Autodesk Fusion 360 part; units mm, degrees
sketch "Sketch2" plane through (0, 0, 0) normal (0, 0, 1) x (1, 0, 0)
  line L0 (-46, 50) -> (126, 50)
  line L1 (130, 46) -> (130, -76)
  line L2 (126, -80) -> (-46, -80)
  line L3 (-50, -76) -> (-50, 46)
  circle A0 centre (-45, 45) radius 2
  line L4 (40, -80) -> (40, 50) construction
  line L5 (-50, -15) -> (130, -15) construction
  arc A1 (-46, 50) -> (-50, 46) centre (-46, 46) ccw
  circle A2 centre (125, 45) radius 2
  arc A3 (130, 46) -> (126, 50) centre (126, 46) ccw
  circle A4 centre (125, -75) radius 2
  arc A5 (126, -80) -> (130, -76) centre (126, -76) ccw
  circle A6 centre (-45, -75) radius 2
  arc A7 (-50, -76) -> (-46, -80) centre (-46, -76) ccw
  point P0 (-50, 50)
  point P1 (130, 50)
  dimension "d3" = 4
  dimension "d4" = 5
  dimension "d5" = 5
  dimension "d6" = 4
  dimension "d63" = 180
  dimension "d64" = 130
extrude "Extrude1" add sketch "Sketch2" along normal blind 6
sketch "Sketch3" plane through (0, 0, 0) normal (0, 0, -1) x (1, 0, 0)
  circle A0 centre (125, 75) radius 2
  circle A1 centre (-45, 75) radius 2
  circle A2 centre (-45, -45) radius 2
  circle A3 centre (125, -45) radius 2
  arc A4 (-50, -46) -> (-46, -50) centre (-46, -46) ccw
  line L0 (-46, -50) -> (126, -50)
  arc A5 (126, -50) -> (130, -46) centre (126, -46) ccw
  line L1 (130, -46) -> (130, 76)
  arc A6 (130, 76) -> (126, 80) centre (126, 76) ccw
  line L2 (126, 80) -> (-46, 80)
  arc A7 (-46, 80) -> (-50, 76) centre (-46, 76) ccw
  line L3 (-50, 76) -> (-50, -46)
  line L4 (40, 80) -> (40, -50) construction
  line L5 (130, 15) -> (-50, 15) construction
  line L6 (119.9494, -39.9494) -> (-39.9494, -39.9494) construction
  line L7 (-39.9494, -39.9494) -> (-39.9494, 69.9494) construction
  line L8 (-39.9494, 69.9494) -> (119.9494, 69.9494) construction
  line L9 (119.9494, 69.9494) -> (119.9494, -39.9494) construction
  line L10 (119.9494, -39.9494) -> (-39.9494, 69.9494) construction
  line L11 (-39.9494, -39.9494) -> (119.9494, 69.9494) construction
  line L12 (108.2459, -41.3839) -> (-28.2459, -41.3839)
  line L13 (-41.3839, -28.2459) -> (-41.3839, 58.2459)
  line L14 (-28.2459, 71.3839) -> (108.2459, 71.3839)
  line L15 (121.3839, 58.2459) -> (121.3839, -28.2459)
  line L16 (95.6336, -23.5438) -> (-41.3839, 71.3839) construction
  line L17 (-38.6963, -33.1786) -> (83.6146, 41.7012) construction
  line L18 (-38.5149, -28.2459) -> (-38.5149, 58.2459)
  line L19 (-28.2459, 68.5149) -> (108.2459, 68.5149)
  line L20 (118.5149, 58.2459) -> (118.5149, -28.2459)
  line L21 (104.513, -28.9713) -> (-38.5149, 68.5149) construction
  line L22 (-36.0332, -30.305) -> (80.8211, 39.3236) construction
  arc A8 (-28.2459, 68.5149) -> (-38.5149, 58.2459) centre (-28.2459, 58.2459) ccw
  arc A9 (-28.2459, 71.3839) -> (-41.3839, 58.2459) centre (-28.2459, 58.2459) ccw
  arc A10 (118.5149, 58.2459) -> (108.2459, 68.5149) centre (108.2459, 58.2459) ccw
  arc A11 (121.3839, 58.2459) -> (108.2459, 71.3839) centre (108.2459, 58.2459) ccw
  arc A12 (-38.5149, -28.2459) -> (-28.2459, -38.5149) centre (-28.2459, -28.2459) ccw
  arc A13 (-41.3839, -28.2459) -> (-28.2459, -41.3839) centre (-28.2459, -28.2459) ccw
  arc A14 (108.2459, -38.5149) -> (118.5149, -28.2459) centre (108.2459, -28.2459) ccw
  arc A15 (108.2459, -41.3839) -> (121.3839, -28.2459) centre (108.2459, -28.2459) ccw
  line L23 (108.2459, -38.5149) -> (-28.2459, -38.5149)
  point P0 (40, 15)
  point P1 (40, 15)
  point P2 (40, 15)
  point P3 (40, 15)
  point P4 (40, 15)
  dimension "d25" = 159.8988
  dimension "d27" = 109.8988
  dimension "d28" = 1.4345
  dimension "d29" = 1.4345
  dimension "d30" = 1.4345
  dimension "d31" = 1.4345
  dimension "d44" = 10.269
  dimension "d45" = 13.138
extrude "Extrude4" add sketch "Sketch3" along normal blind 1.424 contours L12 L13 L14 L15 A9 A11 A13 A15
draft "Draft3" angle 10 neutral plane through (0, 0, -1.424) pull (0, 0, -1) 16 faces at (62.7486, -68.5149, -0.9493) (117.7793, -62.0625, -0.9493) (118.5149, -29.4153, -0.4747) (115.6779, 35.3323, -0.9493) (62.7486, 38.5149, -0.4747) (-32.9514, 37.3734, -0.9493) (-38.5149, -29.4153, -0.9493) (-35.6779, -65.3323, -0.9493) (-41.3839, -0.5847, -0.4747) (-33.1288, 40.4428, -0.9493) (17.2514, 41.3839, -0.9493) (116.3673, 38.5731, -0.9493) (121.3839, -29.4153, -0.9493) (119.6238, -64.8149, -0.9493) (62.7486, -71.3839, -0.9493) (-38.9478, -65.8667, -0.9493)
sketch "Sketch5" plane through (0, 0, -1.424) normal (0, 0, -1) x (1, 0, 0)
  line L0 (-28.2459, 68.5149) -> (108.2459, 68.5149)
  line L1 (118.5149, 58.2459) -> (118.5149, -28.2459)
  line L2 (108.2459, -38.5149) -> (-28.2459, -38.5149)
  line L3 (-38.5149, -28.2459) -> (-38.5149, 58.2459)
  line L4 (108.2459, 71.3839) -> (-28.2459, 71.3839)
  line L5 (-41.3839, 58.2459) -> (-41.3839, -28.2459)
  line L6 (-28.2459, -41.3839) -> (108.2459, -41.3839)
  line L7 (121.3839, -28.2459) -> (121.3839, 58.2459)
  line L8 (40, 71.3839) -> (40, -41.3839) construction
  line L9 (121.3839, 15) -> (-41.3839, 15) construction
  line L10 (119.9494, -39.9494) -> (-39.9494, -39.9494) construction
  line L11 (-39.9494, -39.9494) -> (-39.9494, 69.9494) construction
  line L12 (-39.9494, 69.9494) -> (119.9494, 69.9494) construction
  line L13 (119.9494, 69.9494) -> (119.9494, -39.9494) construction
  line L14 (119.9494, -39.9494) -> (-39.9494, 69.9494) construction
  line L15 (-39.9494, -39.9494) -> (119.9494, 69.9494) construction
  line L16 (108.2459, -40.8839) -> (-28.2459, -40.8839)
  line L17 (-40.8839, -28.2459) -> (-40.8839, 58.2459)
  line L18 (-28.2459, 70.8839) -> (108.2459, 70.8839)
  line L19 (120.8839, 58.2459) -> (120.8839, -28.2459)
  line L20 (98.0985, -25.1411) -> (-40.8839, 70.8839) construction
  line L21 (-40.8839, -40.8839) -> (98.0985, 55.1411) construction
  line L22 (108.2459, -39.0149) -> (-28.2459, -39.0149)
  line L23 (-39.0149, -28.2459) -> (-39.0149, 58.2459)
  line L24 (119.0149, 58.2459) -> (119.0149, -28.2459)
  line L25 (97.1479, -24.0666) -> (-39.0149, 69.0149) construction
  line L26 (-39.0149, -39.0149) -> (97.1479, 54.0666) construction
  arc A0 (118.5149, 58.2459) -> (108.2459, 68.5149) centre (108.2459, 58.2459) ccw
  arc A1 (108.2459, -38.5149) -> (118.5149, -28.2459) centre (108.2459, -28.2459) ccw
  arc A2 (-38.5149, -28.2459) -> (-28.2459, -38.5149) centre (-28.2459, -28.2459) ccw
  arc A3 (-28.2459, 68.5149) -> (-38.5149, 58.2459) centre (-28.2459, 58.2459) ccw
  arc A4 (-41.3839, -28.2459) -> (-28.2459, -41.3839) centre (-28.2459, -28.2459) ccw
  arc A5 (108.2459, -41.3839) -> (121.3839, -28.2459) centre (108.2459, -28.2459) ccw
  arc A6 (121.3839, 58.2459) -> (108.2459, 71.3839) centre (108.2459, 58.2459) ccw
  arc A7 (-28.2459, 71.3839) -> (-41.3839, 58.2459) centre (-28.2459, 58.2459) ccw
  arc A8 (-28.2459, 69.0149) -> (-39.0149, 58.2459) centre (-28.2459, 58.2459) ccw
  arc A9 (-28.2459, 70.8839) -> (-40.8839, 58.2459) centre (-28.2459, 58.2459) ccw
  arc A10 (119.0149, 58.2459) -> (108.2459, 69.0149) centre (108.2459, 58.2459) ccw
  arc A11 (120.8839, 58.2459) -> (108.2459, 70.8839) centre (108.2459, 58.2459) ccw
  line L27 (-28.2459, 69.0149) -> (108.2459, 69.0149)
  arc A12 (108.2459, -39.0149) -> (119.0149, -28.2459) centre (108.2459, -28.2459) ccw
  arc A13 (108.2459, -40.8839) -> (120.8839, -28.2459) centre (108.2459, -28.2459) ccw
  arc A14 (-39.0149, -28.2459) -> (-28.2459, -39.0149) centre (-28.2459, -28.2459) ccw
  arc A15 (-40.8839, -28.2459) -> (-28.2459, -40.8839) centre (-28.2459, -28.2459) ccw
  point P0 (40, 15)
  point P1 (40, 15)
  point P2 (40, 15)
  dimension "d36" = 159.8988
  dimension "d37" = 109.8988
  dimension "d38" = 0.9345
  dimension "d39" = 0.9345
  dimension "d40" = 0.9345
  dimension "d41" = 0.9345
  dimension "d50" = 10.769
  dimension "d51" = 12.638
extrude "Extrude6" cut sketch "Sketch5" against normal blind 1.424 contours L16 L17 L18 L19 A9 A11 A13 A15
extrude "Extrude7" cut 1 faces at (17.2514, 2.7546, 0) along direction (0, 0, 1) blind 0.5
sketch "Sketch6" plane through (0, 0, 0.5) normal (0, 0, -1) x (1, 0, 0)
  line L0 (108.2459, 68.2638) -> (-28.2459, 68.2638)
  arc A0 (-28.2459, 68.2638) -> (-38.2638, 58.2459) centre (-28.2459, 58.2459) ccw
  line L1 (-38.2638, 58.2459) -> (-38.2638, -28.2459)
  arc A1 (-38.2638, -28.2459) -> (-28.2459, -38.2638) centre (-28.2459, -28.2459) ccw
  line L2 (-28.2459, -38.2638) -> (108.2459, -38.2638)
  arc A2 (108.2459, -38.2638) -> (118.2638, -28.2459) centre (108.2459, -28.2459) ccw
  line L3 (118.2638, -28.2459) -> (118.2638, 58.2459)
  arc A3 (118.2638, 58.2459) -> (108.2459, 68.2638) centre (108.2459, 58.2459) ccw
  line L4 (40, 68.2638) -> (40, -38.2638) construction
  line L5 (-38.2638, 15) -> (118.2638, 15) construction
  line L6 (96, -27.5) -> (-16, -27.5)
  line L7 (-20, -23.5) -> (-20, 53.5)
  line L8 (-16, 57.5) -> (96, 57.5)
  line L9 (100, 53.5) -> (100, -23.5)
  line L10 (100, -27.5) -> (-20, 57.5) construction
  line L11 (-20, -27.5) -> (100, 57.5) construction
  arc A4 (-16, 57.5) -> (-20, 53.5) centre (-16, 53.5) ccw
  arc A5 (100, 53.5) -> (96, 57.5) centre (96, 53.5) ccw
  arc A6 (96, -27.5) -> (100, -23.5) centre (96, -23.5) ccw
  arc A7 (-20, -23.5) -> (-16, -27.5) centre (-16, -23.5) ccw
  point P0 (40, 15)
  dimension "d58" = 120
  dimension "d59" = 85
  dimension "d68" = 4
  dimension "d69" = 4
  dimension "d70" = 4
  dimension "d71" = 4
extrude "Extrude8" cut sketch "Sketch6" against normal blind 1.1 contours L6 L7 L8 L9 A4 A5 A6 A7
sketch "Sketch7" plane through (0, 0, 1.6) normal (0, 0, -1) x (1, 0, 0)
  line L0 (96, 57.5) -> (-16, 57.5)
  line L1 (-20, 53.5) -> (-20, -23.5)
  line L2 (-16, -27.5) -> (96, -27.5)
  line L3 (100, -23.5) -> (100, 53.5)
  line L4 (40, 57.5) -> (40, -27.5) construction
  line L5 (100, 15) -> (-20, 15) construction
  line L6 (91, -22.5) -> (-11, -22.5)
  line L7 (-15, -18.5) -> (-15, 48.5)
  line L8 (-11, 52.5) -> (91, 52.5)
  line L9 (95, 48.5) -> (95, -18.5)
  line L10 (95, -22.5) -> (-15, 52.5) construction
  line L11 (-15, -22.5) -> (95, 52.5) construction
  arc A0 (-16, 57.5) -> (-20, 53.5) centre (-16, 53.5) ccw
  arc A1 (-20, -23.5) -> (-16, -27.5) centre (-16, -23.5) ccw
  arc A2 (96, -27.5) -> (100, -23.5) centre (96, -23.5) ccw
  arc A3 (100, 53.5) -> (96, 57.5) centre (96, 53.5) ccw
  arc A4 (-11, 52.5) -> (-15, 48.5) centre (-11, 48.5) ccw
  arc A5 (95, 48.5) -> (91, 52.5) centre (91, 48.5) ccw
  arc A6 (91, -22.5) -> (95, -18.5) centre (91, -18.5) ccw
  arc A7 (-15, -18.5) -> (-11, -22.5) centre (-11, -18.5) ccw
  point P0 (40, 15)
  dimension "d62" = 110
  dimension "d65" = 75
  dimension "d72" = 4
  dimension "d73" = 4
  dimension "d74" = 4
  dimension "d75" = 4
extrude "Extrude9" cut sketch "Sketch7" against normal blind 8.4 contours L6 L7 L8 L9 A4 A5 A6 A7
equation "ORingDiameter = 1.78 mm"
equation "ORingInnerDiameter = 170 mm"
equation "d25 = ( ORingPerimeter - 100 mm ) / 4 + 50 mm"
equation "ORingPerimeter = 2 * 3.1412 * ( ( ORingInnerDiameter / 2 ) + ORingDiameter / 2 )"
equation "d27 = ( ORingPerimeter - 100 mm ) / 4"
equation "d28 = ( ( ORingDiameter * 1.05 ) / 2 ) + 0.5 mm"
equation "d29 = ( ( ORingDiameter * 1.05 ) / 2 ) + 0.5 mm"
equation "d30 = ( ( ORingDiameter * 1.05 ) / 2 ) + 0.5 mm"
equation "d31 = ( ( ORingDiameter * 1.05 ) / 2 ) + 0.5 mm"
equation "d32 = ORingDiameter * 0.8"
equation "d36 = ( ORingPerimeter - 100 mm ) / 4 + 50 mm"
equation "d37 = ( ORingPerimeter - 100 mm ) / 4"
equation "d38 = ( ORingDiameter * 1.05 ) / 2"
equation "d39 = ( ORingDiameter * 1.05 ) / 2"
equation "d40 = ( ORingDiameter * 1.05 ) / 2"
equation "d41 = ( ORingDiameter * 1.05 ) / 2"
equation "d44 = ( ORingDiameter ) * 6 + ORingDiameter * 0.05 - 0.5 mm"
equation "d45 = ( ORingDiameter ) * 6 + ( ORingDiameter * 1.1 ) + 0.5 mm"
equation "d50 = ( ORingDiameter ) * 6 + ORingDiameter * 0.05 - 0.0 mm"
equation "d51 = ( ORingDiameter ) * 6 + ORingDiameter * 1.1 + 0 mm"
equation "d52 = -( ORingDiameter * 0.8 )"
equation "PanelWidth = 85 mm"
equation "PanelLength = 120 mm"
equation "d58 = PanelLength"
equation "d59 = PanelWidth"
equation "d62 = PanelLength - 10 mm"
equation "d65 = PanelWidth - 10 mm"
Read the model definition and answer for the solid it produces. Units are mm, in the model's axes. A direction names the side the tool comes from. Give positions to 0.01 mm unless a question says otherwise; leave off trailing zeros.
(1) Given pin 1 (1.1 mm diameter, centred on x = 13.5, z = -1, fed in from +Y); pin 2 (6.5 mm diameter, centred on x = 125, y = 45, fed in from -Z); pin 3 (1.1 mm diameter, centred on x = 71.5, z = -0.5, fed in from +Y); pin 4 (1.5 mm diameter, centred on x = -13.5, y = 12.5, fed in from +Z), each flat-ended and moving along its own axis, determine where each tip first touches the part or whether it passes through.
(2) For a pull along Y with two mould halves and no side action, classify faces 1 (the flat face through (-15, -15, 4)), 2 (the conical face through (-37.7, -67.5, -0.9)), 3 (the cylindrical face through (-18.859, 26.297, 1.042)), 4 (the flat face through (33, -72, 0)) as released by +Y, released by -Y, zero draft, split by the parting line, or undercut.
(3) Straight lines are drawn through the part: L1, parallel to Y at x = -45, z = 3.95; L2, parallel to Y at x = 38, z = 1; L3, parallel to X at y = -7.5, z = 4.75. For each, find the intervals that lie inside material, in ascending order.
(4) For faces 5 (the conical face through (117.7, 37.5, -0.9)), 6 (the cylindrical face through (115.78, 35.94, -0.72)), 7 (the cylindrical face through (93.797, 21.359, 3.769)), determine the directions among +Z, -Z, +X, -X, +Y, -Y from which every point of the face is accessible in a straight line to the end or side of a thin tool.
Result sheet:
1. pin 1: stops at y = 41.56
1. pin 2: stops at z = 0
1. pin 3: stops at y = 50
1. pin 4: passes through
2. face 1: undercut
2. face 2: released by -Y
2. face 3: undercut
2. face 4: zero draft
3. L1: y = -80 to -77, -73 to 43, 47 to 50
3. L2: y = -80 to -57.5, 27.5 to 50
3. L3: x = -50 to -15, 95 to 130
4. face 5: -Z, +X, +Y
4. face 6: -Z
4. face 7: +Z, -Z
